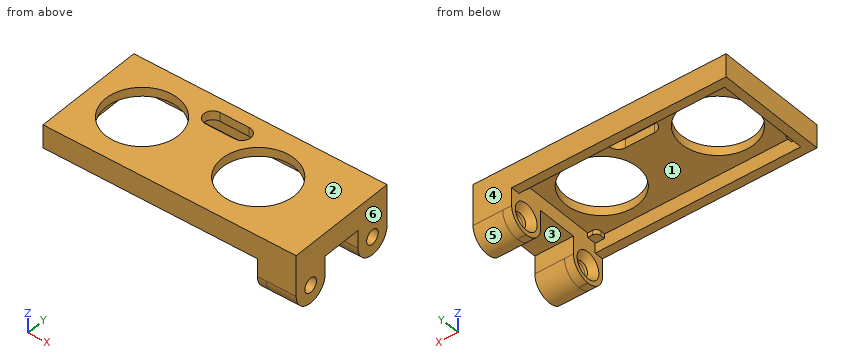
Autodesk Inventor part; units mm, degrees
ref_plane "РабПлоскость1" through (25, 2, 0) normal (1, 0, 0) x (0, 0, -1)
ref_plane "РабПлоскость2" through (2, 12.5, 0) normal (0, -1, 0) x (1, 0, 0)
ref_plane "РабПлоскость6" through (0, 12.5, 5.2) normal (0, 1, 0) x (1, 0, 0)
sketch "Эскиз1" plane through (0, 0, 0) normal (0, 0, 1) x (1, 0, 0)
  line L0 (0, 0) -> (50, 0)
  line L1 (50, 0) -> (50, 25)
  line L2 (50, 25) -> (0, 25)
  line L3 (0, 25) -> (0, 0)
  dimension "d0" = 50
  dimension "d1" = 25
extrude "Выдавливание1" add sketch "Эскиз1" along normal blind 5.2
shell "Оболочка1" thickness 2 removed faces 1 at (16.6667, 16.6667, 0)
sketch "Эскиз2" plane through (0, 0, 5.2) normal (0, 0, 1) x (1, 0, 0)
  line L0 (50, 25) -> (0, 25)
  line L1 (25, 25) -> (25, 0)
  line L2 (0, 0) -> (50, 0)
  line L3 (25, 12.5) -> (12, 12.5)
  line L4 (0, 25) -> (0, 0)
  circle A0 centre (12, 12.5) radius 8.1
  circle A1 centre (38, 12.5) radius 8.1
  line L5 (25, 25) -> (25, 20)
  line L6 (21.75, 20) -> (28.25, 20) construction
  line L7 (21.75, 18) -> (28.25, 18)
  line L8 (28.25, 22) -> (21.75, 22)
  arc A2 (21.75, 22) -> (21.75, 18) centre (21.75, 20) ccw
  arc A3 (28.25, 18) -> (28.25, 22) centre (28.25, 20) ccw
  point P0 (25, 18)
  point P1 (25, 22)
  dimension "d5" = 13
  dimension "d6" = 16.2
  dimension "d9" = 5
  dimension "d10" = 3.25
  dimension "d11" = 4
extrude "Выдавливание2" cut sketch "Эскиз2" against normal through all contours L8 A3 L7 L1 | L1 L7 A2 L8 | A0 | A1
sketch "Эскиз5" plane through (48, 23, 3.2) normal (0, 0, -1) x (-1, 0, 0)
  line L0 (0, 0) -> (1.05, 0)
  line L1 (0, 0) -> (46, 0)
  line L2 (1.05, 0) -> (1.05, -1.05)
  circle A0 centre (1.05, -1.05) radius 1.05
  line L3 (2.1, -2.1) -> (0, -2.1)
  line L4 (0, -2.1) -> (0, 0)
  line L5 (0, 0) -> (2.1, 0)
  line L6 (2.1, 0) -> (2.1, -2.1)
  line L7 (2.1, -2.1) -> (0, 0) construction
  line L8 (0, -2.1) -> (2.1, 0) construction
  point P0 (48, -23)
  point P1 (1.05, -2.1)
  point P2 (2.1, -1.05)
  dimension "d17" = 1.05
  dimension "d18" = 1.05
extrude "Выдавливание4" add sketch "Эскиз5" along normal blind 1 contours L0 A0 L4 | L1 L6 A0 | A0 | A0 L3 L4
ref_plane "РабПлоскость1" through (25, 2, 0) normal (1, 0, 0) x (0, 0, -1)
ref_plane "РабПлоскость2" through (2, 12.5, 0) normal (0, -1, 0) x (1, 0, 0)
mirror "Зеркальное отражение1" about plane through (2, 12.5, 0) normal (0, -1, 0) of "Выдавливание4"
mirror "Зеркальное отражение2" about plane through (25, 2, 0) normal (1, 0, 0) of "Выдавливание4", "Зеркальное отражение1"
sketch "Эскиз11" plane through (50, 25, 5.2) normal (1, 0, 0) x (0, 0, -1)
  line L0 (5.2, 0) -> (13.2, 0)
  line L1 (13.2, 0) -> (13.2, -8)
  line L2 (13.2, -8) -> (5.2, -8)
  line L3 (5.2, -8) -> (5.2, 0)
  point P0 (5.2, -25)
  dimension "d53" = 8
  dimension "d54" = 8
extrude "Выдавливание8" add sketch "Эскиз11" against normal blind 2
sketch "Эскиз12" plane through (48, 23, 0) normal (-1, 0, 0) x (0, 0, 1)
  line L0 (-8, -6) -> (0, -6)
  line L1 (-4, -6) -> (-4, 2)
  point P0 (0, -23)
  point P1 (-4, -2)
hole "Отверстие3" at (48, 21, -4) direction (1, 0, 0) diameter 3.2 end through all countersink diameter 6 countersink angle 90
ref_plane "РабПлоскость6" through (0, 12.5, 5.2) normal (0, 1, 0) x (1, 0, 0)
mirror "Зеркальное отражение5" about plane through (0, 12.5, 5.2) normal (0, 1, 0) of "Выдавливание8", "Отверстие3"
fillet "Сопряжение3" radius 4 4 edges at (49, 25, -8) (49, 17, -8) (49, 0, -8) (49, 8, -8)
sketch "Эскиз13" plane through (50, 0, 5.2) normal (1, 0, 0) x (0, 0, -1)
  arc A0 (9.2, 0) -> (9.2, 8) centre (9.2, 4) ccw
  line L0 (5.2, 8) -> (9.2, 8)
  line L1 (5.2, 8) -> (5.2, 17)
  line L2 (5.2, 17) -> (9.2, 17)
  arc A1 (9.2, 17) -> (9.2, 25) centre (9.2, 21) ccw
  line L3 (9.2, 25) -> (0, 25)
  line L4 (0, 0) -> (0, 25)
  line L5 (9.2, 0) -> (0, 0)
  circle A2 centre (9.2, 21) radius 1.6
  circle A3 centre (9.2, 4) radius 1.6
  point P0 (5.2, 0)
extrude "Выдавливание9" add sketch "Эскиз13" along normal blind 6.65
properties part number "Крепление ультрасоника вертикальная"
For this review, take the finished solid that the model builds, in its own axes (mm). Face numbers are marked on the shaded views. A direction names the side the tool comes from. Coordinates: 2 decimals unless noted, no trailing zeros. Loops run counter-clockwise (first coordinate to the right, second up) from the corner with the lowest first, then second, coordinate; pieces in that order, holes last. Notation, with made-up numbers: (-11.5, 2.5) -> (27.5, 2.5) arc R13 cw to (27.5, 8.5) -> close; hole circle Ø8 at (87, 35.5). An arc over 180 degrees is marked (long way). Return JSON: item names as keys, results as strings. Group by question number.
(1) For pin 1 Ø9.5 at (x, y) = (12, 12.5) entering from -Z; pin 2 Ø1.7 at (x, y) = (3.5, 21.5) entering from -Z; pin 3 Ø5 at (y, z) = (3, -4) entering from -X; pin 4 Ø2.5 at (x, y) = (3, 3.5) entering from -Z, all flat-tipped, find the tip position at first contact; note any pin that passes through.
(2) Consider section D-D, the plane y = 20. Count the separate pieces of the cut face and the enclosed holes in it, plus the area to 3 significant figures.
(3) Consider section A-A, the plane y = 12.5. Give the boundary of the cut face in (x, z).
(4) Consider section B-B, the plane x = 25. Give the boundary of the cut face in (y, z).
(5) Consider section C-C, the plane x = 31.5. Give the boundary of the cut face in (y, z), plus the area to 3 significant figures.
(6) Mouldability with a two-part tool opening along Y and no side actions: class the marked faces 4, 5 and 6 as pulls with the +Y half, pulls with the -Y half, needs draft (parallel to the pull), parting line crosses it, or undercut.
(7) To check wall thickness, follow L1, parallel to Y at x = 49.5, z = -4; L2, parallel to X at y = 2.5, z = 1.75; L3, parallel to Z at x = 49.75, y = 4. State the ranges of each line that lie inside material, in increasing order.
(8) Tool access review of the marked faces 1, 2 and 3: name each direction out of +Z, -Z, +X, -X, +Y, -Y from which nothing blocks a thin tool from reaching the whole face with its end or side.
Results below:
{
 "1": {"pin 1": "passes through", "pin 2": "stops at z = 2.2", "pin 3": "stops at x = 48", "pin 4": "stops at z = 0"},
 "2": {"separate pieces": "5", "enclosed holes": "0", "area": "146 mm2"},
 "3": {"outline": "(0, 0) -> (2, 0) -> (2, 3.2) -> (3.9, 3.2) -> (3.9, 5.2) -> (0, 5.2) -> close; (20.1, 3.2) -> (29.9, 3.2) -> (29.9, 5.2) -> (20.1, 5.2) -> close; (46.1, 3.2) -> (48, 3.2) -> (48, 0) -> (56.65, 0) -> (56.65, 5.2) -> (46.1, 5.2) -> close"},
 "4": {"outline": "(0, 0) -> (2, 0) -> (2, 3.2) -> (18, 3.2) -> (18, 5.2) -> (0, 5.2) -> close; (22, 3.2) -> (23, 3.2) -> (23, 0) -> (25, 0) -> (25, 5.2) -> (22, 5.2) -> close"},
 "5": {"outline": "(0, 0) -> (2, 0) -> (2, 3.2) -> (7.67, 3.2) -> (7.67, 5.2) -> (0, 5.2) -> close; (17.33, 3.2) -> (23, 3.2) -> (23, 0) -> (25, 0) -> (25, 5.2) -> (17.33, 5.2) -> close", "area": "43.5 mm2"},
 "6": {"face 4": "pulls with the +Y half", "face 5": "undercut", "face 6": "needs draft"},
 "7": {"L1": "y = 0 to 2.4, 5.6 to 8, 17 to 19.4, 22.6 to 25", "L2": "x = 0 to 2, 48 to 56.65", "L3": "z = -8 to -5.6, -2.4 to 5.2"},
 "8": {"face 1": "-Z", "face 2": "+Z, +X, -X, +Y, -Y", "face 3": "-Z, +X, -X"}
}
